Build history of the part. All positions in model axes, mm. A direction names the side the tool comes from. Round coordinates to 2 decimals unless told otherwise and drop trailing zeros. Loops run counter-clockwise (first coordinate to the right, second up) from the corner with the lowest first, then second, coordinate; pieces in that order, holes last. Notation, with made-up numbers: (86, 30.5) - (138, 30.5) arc R9 ccw to (138, 37.5) - close; hole circle Ø9 at (59, 25.5). An arc over 180 degrees is marked (long way). Put each result on its own line as item: value. Start each with the question number.
from build123d import *

# Parameters (mm, degrees)
F0_W     = 76.2
F0_H     = 76.2
F1_DEPTH = 3.175
F2_W     = 3.175
F2_H     = 3.175
F2_W_2   = 22.225
F2_H_2   = 22.225
F3_DEPTH = 25.4


with BuildPart() as f1:
    # F0 (on Top) → F1 (new body)
    with BuildSketch(Plane.XY):
        Rectangle(F0_W, F0_H)
    extrude(amount=F1_DEPTH)

    # F2 (on face) → F3 (cut)
    with BuildSketch(Plane.XY.offset(3.175)):
        with Locations((-36.5125, 36.5125)):
            Rectangle(F2_W, F2_H)
        with Locations((-23.8125, 36.5125)):
            Rectangle(F2_W_2, F2_H)
        with Locations((-36.5125, 23.8125)):
            Rectangle(F2_W, F2_H_2)
        with Locations((-36.5125, -23.8125)):
            Rectangle(F2_W, F2_H_2)
        with Locations((-36.5125, -36.5125)):
            Rectangle(F2_W, F2_H)
        with Locations((-23.8125, -36.5125)):
            Rectangle(F2_W_2, F2_H)
        with Locations((23.8125, -36.5125)):
            Rectangle(F2_W_2, F2_H)
        with Locations((36.5125, -23.8125)):
            Rectangle(F2_W, F2_H_2)
        with Locations((36.5125, -36.5125)):
            Rectangle(F2_W, F2_H)
        with Locations((36.5125, 23.8125)):
            Rectangle(F2_W, F2_H_2)
        with Locations((23.8125, 36.5125)):
            Rectangle(F2_W_2, F2_H)
        with Locations((36.5125, 36.5125)):
            Rectangle(F2_W, F2_H)
    extrude(amount=-F3_DEPTH, mode=Mode.SUBTRACT)


solid = f1.part
Item 1: Slice it at B-B (y = -22). Give the cut face in (x, z) (3 decimals), plus the area to 3 significant figures.
Item 2: Which spindle directions (+Z, -Z, +X, -X, +Y, -Y) get a long thin tool onto all of the face, cutting with end or side? Do faces 1 (the flat face through (-24, 34.925, 2)), 2 (the flat face through (34.925, 24, 2)), 3 (the flat face through (34.925, -24, 2)), 4 (the flat face through (-34.925, -24, 2)), 5 (the flat face through (0, -38.1, 2)). Say none if no direction does.
Item 3: Drill centre line: probe 1 along Y at (x, z) = (34.5, 1.4) (3 decimals). Where is it in solid material? Low to high. Write a range as [from, to].
Item 4: Slice it at A-A (z = 2.3). Give the cut face in (x, y) (3 decimals).
Item 5: Drop flat-ended pins along their axis: pin 1 Ø10 at (x, y) = (-14, -27.5) entering from -Z; pin 2 Ø1.6 at (y, z) = (-36, 1.5) entering from +X; pin 3 Ø1 at (x, z) = (36.5, 1) entering from -Y; pin 4 Ø1 at (y, z) = (-19, 2) entering from +X (3 decimals). Give the stop position or say it passes through.
Computed values:
1. outline: (-34.925, 0) - (34.925, 0) - (34.925, 3.175) - (-34.925, 3.175) - close
1. area: 222 mm^2
2. face 1: +Z, -Z, -X, +Y
2. face 2: +Z, -Z, +X, +Y
2. face 3: +Z, -Z, +X, -Y
2. face 4: +Z, -Z, -X, -Y
2. face 5: +Z, -Z, +X, -X, -Y
3. probe 1: y = [-34.925, 34.925]
4. outline: (-38.1, -12.7) - (-34.925, -12.7) - (-34.925, -34.925) - (-12.7, -34.925) - (-12.7, -38.1) - (12.7, -38.1) - (12.7, -34.925) - (34.925, -34.925) - (34.925, -12.7) - (38.1, -12.7) - (38.1, 12.7) - (34.925, 12.7) - (34.925, 34.925) - (12.7, 34.925) - (12.7, 38.1) - (-12.7, 38.1) - (-12.7, 34.925) - (-34.925, 34.925) - (-34.925, 12.7) - (-38.1, 12.7) - close
5. pin 1: stops at z = 0
5. pin 2: stops at x = 12.7
5. pin 3: stops at y = -12.7
5. pin 4: stops at x = 34.925
